Part model, mm, in its own coordinate system. Round coordinates to 2 decimals unless told otherwise and drop trailing zeros. Write each loop counter-clockwise with the first axis right and the second up, starting at its lowest first coordinate (ties: lowest second). Pieces come first, ordered by that corner, then holes. Notation, with made-up numbers: M -26.5,34 L 31.5,34 A25 ccw 31.5,70 Z; hole C -16,-3 d7. An arc over 180 degrees is marked long. Answer as a JSON object with one key per item and string values. Group by question number.
1. Band-saw the part on A-A, the plane y = -239. Write the cut outline in (x, z), plus the area to 3 significant figures.
2. Drill centre lines: line 1 (Y direction, x = 0, z = 1.4); line 2 (Y direction, x = -6, z = -2.5); line 3 (Z direction, x = 1.5, y = -407.5). Where is each one in solid material? Low to high. Write a range as from..to.
3. Drop flat-ended pins along their axis: pin 1 (5 mm diameter, centred on x = -1.5, y = -212.5, fed in from -Z); pin 2 (5.5 mm diameter, centred on y = -327.5, z = 2, fed in from +X); pin 3 (1 mm diameter, centred on x = 2.5, y = -243.5, fed in from +Z). Give the stop position or say it passes through.
from build123d import *

# Parameters (mm, degrees)
SKETCH1_W           = 6
SKETCH1_H           = 500
SKETCH1_R           = 2
BOSS_EXTRUDE1_DEPTH = 5
SKETCH2_W           = 30
SKETCH2_H           = 30
BOSS_EXTRUDE2_DEPTH = 100
FILLET1_R           = 10


with BuildPart() as part:
    # Sketch1 → Boss-Extrude1 (new body)
    with BuildSketch(Plane.XY):
        with Locations((0, -247)):
            Rectangle(SKETCH1_W, SKETCH1_H)
        Circle(SKETCH1_R, mode=Mode.SUBTRACT)
    extrude(amount=BOSS_EXTRUDE1_DEPTH)

    # Sketch2 → Boss-Extrude2 (add)
    with BuildSketch(Plane.XZ.offset(497)):
        with Locations((0, 2.5)):
            Rectangle(SKETCH2_W, SKETCH2_H)
    extrude(amount=BOSS_EXTRUDE2_DEPTH)

    # Fillet1
    fillet1_edges = [part.edges().sort_by_distance(p)[0] for p in [
        (15, -547, -12.5),
        (15, -547, 17.5),
        (-15, -547, 17.5),
        (-15, -547, -12.5),
    ]]
    fillet(fillet1_edges, radius=FILLET1_R)


solid = part.part
Worked answers:
{
 "1": {"outline": "M -3,0 L 3,0 L 3,5 L -3,5 Z", "area": "30.0 mm^2"},
 "2": {"line 1": "y = -597..-2, 2..3", "line 2": "y = -597..-497", "line 3": "z = 0..5"},
 "3": {"pin 1": "stops at z = 0", "pin 2": "stops at x = 3", "pin 3": "stops at z = 5"}
}
